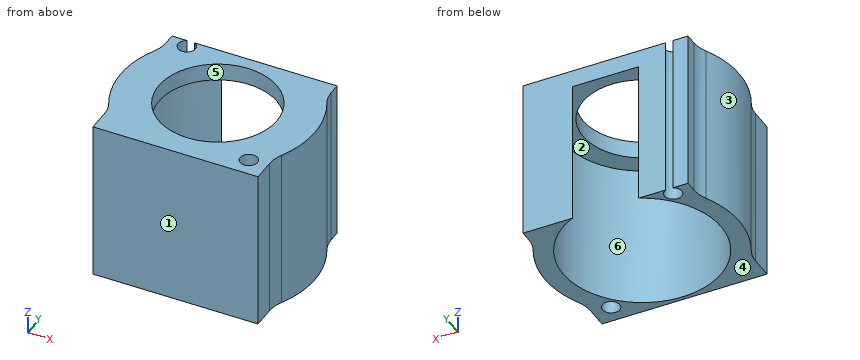
```python
from build123d import *

# Parameters (mm, degrees)
SKETCH1_W               = 47.625
SKETCH1_H               = 47.625
SKETCH1_R               = 22.75
SKETCH1_R_2             = 2.4892
BOSS_EXTRUDE1_DEPTH     = 46.8
CUT_EXTRUDE1_DEPTH      = 58.656832314
CUT_EXTRUDE1_DEPTH_BACK = 58.656832314
SKETCH2_W               = 47.625
SKETCH2_H               = 3.175
BOSS_EXTRUDE2_DEPTH     = 46.8
FILLET1_R               = 10
BOSS_EXTRUDE3_START     = -5
SKETCH4_R               = 17
BOSS_EXTRUDE3_DEPTH     = 5


with BuildPart() as part:
    # Sketch1 → Boss-Extrude1 (new body)
    with BuildSketch(Plane.XY):
        Rectangle(SKETCH1_W, SKETCH1_H)
        Circle(SKETCH1_R, mode=Mode.SUBTRACT)
        with Locations((-18.384776311, 18.384776311)):
            Circle(SKETCH1_R_2, mode=Mode.SUBTRACT)
        with Locations((18.384776311, -18.384776311)):
            Circle(SKETCH1_R_2, mode=Mode.SUBTRACT)
    extrude(amount=BOSS_EXTRUDE1_DEPTH)

    # Sketch2 → Cut-Extrude1 (cut, two sides: drawn at the far end of the back side and taken through both)
    with BuildSketch(Plane.XY.offset(46.8).offset(-CUT_EXTRUDE1_DEPTH_BACK)):
        with Locations((0, 22.225)):
            Rectangle(SKETCH2_W, SKETCH2_H)
    extrude(amount=CUT_EXTRUDE1_DEPTH + CUT_EXTRUDE1_DEPTH_BACK, mode=Mode.SUBTRACT)

    # Sketch3 → Boss-Extrude2 (add)
    with BuildSketch(Plane.XY.offset(46.8)):
        with BuildLine():
            Line((23.8125, -14.729726533), (23.8125, 14.729726533))
            ThreePointArc((23.8125, 14.729726533), (28, 0), (23.8125, -14.729726533))
        make_face()
        with BuildLine():
            Line((-23.8125, 14.729726533), (-23.8125, -14.729726533))
            ThreePointArc((-23.8125, -14.729726533), (-28, 0), (-23.8125, 14.729726533))
        make_face()
    extrude(amount=-BOSS_EXTRUDE2_DEPTH)

    # Fillet1
    fillet1_edges = [part.edges().sort_by_distance(p)[0] for p in [
        (-23.8125, -14.729726533, 23.4),
        (-23.8125, 14.729726533, 23.4),
        (23.8125, 14.729726533, 23.4),
        (23.8125, -14.729726533, 23.4),
    ]]
    fillet(fillet1_edges, radius=FILLET1_R)

    # Sketch4 → Boss-Extrude3 (add)
    with BuildSketch(Plane.XY.offset(46.8).offset(BOSS_EXTRUDE3_START)):
        with BuildLine():
            Line((-9.573718909, 20.6375), (9.573718909, 20.6375))
            ThreePointArc((9.573718909, 20.6375), (0, -22.75), (-9.573718909, 20.6375))
        make_face()
        Circle(SKETCH4_R, mode=Mode.SUBTRACT)
    extrude(amount=BOSS_EXTRUDE3_DEPTH)


solid = part.part
```
Geometry check sheet. Reference: the model listing, model coordinates, mm. Face numbers are marked on the shaded views. A direction names the side the tool comes from. Round coordinates to 2 decimals unless told otherwise and drop trailing zeros. Order: outer loops, then holes, each group sorted by start corner. A loop starts at its lowest first (then second) coordinate and runs counter-clockwise, first axis right, second up. Notation, with made-up numbers: (37, 22) - (91, 22) arc R30 ccw to (91, 48) - close; hole circle Ø2 at (-19, 5.25). An arc over 180 degrees is marked (long way). Use a Markdown table: item, result. Add a question column.
1) Thickness scan on line 1 along X through (y, z) = (0, 33); line 2 along Y through (x, z) = (0, 44); line 3 along X through (y, z) = (16.5, 9.5). Record the ranges inside material, lowest first.
2) Section check C-C (z = 23.5). Record the cut outline in (x, y).
3) Mould release check, pull along X, two halves, no side actions. Record for the marked faces 3, 4, 5 and 6: released by +X, released by -X, zero draft, split by the parting line, or undercut.
4) Set-up check for the marked faces 1 and 2: record each of +Z, -Z, +X, -X, +Y, -Y from which the full face is reachable in a straight line by a thin tool's end or side.
5) Gauge pin test, flat ends, axial feed: P1, Ø1.9, axis at y = -21, z = 25.5, coming from the -X side; P2, Ø3, axis at x = -18.38, y = 18.38, coming from the -Z side; P3, Ø3, axis at y = -22, z = 15.5, coming from the +X side; P4, Ø10, axis at y = -10, z = 32, coming from the -X side. Record the tip position at first contact, or that the pin passes through.
6) Section check A-A (x = 0). Record the cut outline in (y, z).
7) Section check D-D (x = 11). Record the cut outline in (y, z).
8) Section check B-B (y = 0). Record the cut outline in (x, z), then the cut area to 3 significant figures.
Established:
| question | item | result |
|---|---|---|
| 1 | line 1 | -28 to -22.75, 22.75 to 28 |
| 1 | line 2 | -23.81 to -17, 17 to 20.64 |
| 1 | line 3 | -23.85 to -20.01, -16.76 to -15.66, 15.66 to 23.85 |
| 2 | outline | (-24.91, -12.78) arc R10 cw to (-23.81, -17.34) - (-23.81, -23.81) - (23.81, -23.81) - (23.81, -17.34) arc R10 cw to (24.91, -12.78) arc R28 ccw to (24.91, 12.78) arc R10 cw to (23.81, 17.34) - (23.81, 20.64) - (9.57, 20.64) arc R22.75 cw (long way) to (-9.57, 20.64) - (-17.33, 20.64) arc R2.49 cw (long way) to (-19.44, 20.64) - (-23.81, 20.64) - (-23.81, 17.34) arc R10 cw to (-24.91, 12.78) arc R28 ccw to start; hole circle Ø4.98 at (18.38, -18.38) |
| 3 | face 3 | released by -X |
| 3 | face 4 | zero draft |
| 3 | face 5 | undercut |
| 3 | face 6 | undercut |
| 4 | face 1 | +Z, -Z, +X, -X, -Y |
| 4 | face 2 | -Z |
| 5 | P1 | x = -23.81 |
| 5 | P2 | through |
| 5 | P3 | x = 23.81 |
| 5 | P4 | x = -27.55 |
| 6 | outline | (-23.81, 0) - (-22.75, 0) - (-22.75, 41.8) - (-17, 41.8) - (-17, 46.8) - (-23.81, 46.8) - close; (17, 41.8) - (20.64, 41.8) - (20.64, 46.8) - (17, 46.8) - close |
| 7 | outline | (-23.81, 0) - (-19.91, 0) - (-19.91, 41.8) - (-12.96, 41.8) - (-12.96, 46.8) - (-23.81, 46.8) - close; (12.96, 41.8) - (19.91, 41.8) - (19.91, 0) - (20.64, 0) - (20.64, 46.8) - (12.96, 46.8) - close |
| 8 | outline | (-28, 0) - (-22.75, 0) - (-22.75, 41.8) - (-17, 41.8) - (-17, 46.8) - (-28, 46.8) - close; (17, 41.8) - (22.75, 41.8) - (22.75, 0) - (28, 0) - (28, 46.8) - (17, 46.8) - close |
| 8 | area | 549 mm2 |
